from build123d import *

# Parameters (mm, degrees)
SK_PATILLA_R   = 5.1
SK_PATILLA_R_2 = 5
PATILLA_DEPTH  = 8


with BuildPart() as part:
    # Sk_Patilla → Patilla (new body)
    with BuildSketch(Plane.XY.offset(44.4)):
        with BuildLine():
            Line((3.547963542, -28.972606971), (11.45755625, -3.567128365))
            ThreePointArc((11.45755625, -3.567128365), (2.69831408, 11.692694348), (-11.862050632, 1.814319377))
            Line((-11.862050632, 1.814319377), (-15.885042193, -24.488067186))
            ThreePointArc((-15.885042193, -24.488067186), (-8.248595067, -35.743911957), (3.547963542, -28.972606971))
        make_face()
        Circle(SK_PATILLA_R, mode=Mode.SUBTRACT)
        with Locations((-6, -26)):
            Circle(SK_PATILLA_R_2, mode=Mode.SUBTRACT)
    extrude(amount=PATILLA_DEPTH)


solid = part.part
Model file for the job. Use its own axes, mm. Give positions to 0.01 mm unless a question says otherwise; leave off trailing zeros. Loops run counter-clockwise (first coordinate to the right, second up) from the corner with the lowest first, then second, coordinate; pieces in that order, holes last.
Item 1: Slice it at C-C (z = 49.25). Write the cut outline in (x, y), plus the area to 3 significant figures.
Check values:
outline: (-15.89, -24.49) arc R10 ccw to (3.55, -28.97) - (11.46, -3.57) arc R12 ccw (long way) to (-11.86, 1.81) - close; hole circle Ø10 at (-6, -26); hole circle Ø10.2 at (0, 0)
area: 812 mm2
Item 2: Drop a flat-ended pin along its axis: P1, Ø1.5, axis at y = 5.5, z = 49.5, coming from the -X side. Give the stop position or say it passes through.
Check values:
P1: stops at x = -11.02
Item 3: Slice it at D-D (y = -12.5). Write the cut outline in (x, z).
Check values:
outline: (-14.05, 44.4) - (8.68, 44.4) - (8.68, 52.4) - (-14.05, 52.4) - close
Item 4: Drill centre lines: line 1 along Y through (x, z) = (-1.5, 50.25); line 2 along Y through (x, z) = (-6, 49.75); line 3 along Y through (x, z) = (0, 48.75). Where is each one in solid material? Low to high.
Check values:
line 1: y = -34.93 to -28.18, -23.82 to -4.87, 4.87 to 11.91
line 2: y = -36 to -31, -21 to 10.39
line 3: y = -34 to -5.1, 5.1 to 12
Item 5: Mould opens along X. For faces 1 (the face through (-7.08, -30.88, 48.34)), 2 (the face through (-2, -12, 52.4)), 3 (the face through (7.447, -16.448, 48.344)) say: +X half, -X half, draft (parallel to the pull), parting line (faces both ways), or undercut.
Check values:
face 1: undercut
face 2: draft
face 3: +X half
Item 6: Slice it at A-A (x = 0). Write the cut outline in (y, z).
Check values:
outline: (-34, 44.4) - (-5.1, 44.4) - (-5.1, 52.4) - (-34, 52.4) - close; (5.1, 44.4) - (12, 44.4) - (12, 52.4) - (5.1, 52.4) - close
Item 7: Slice it at B-B (y = 0). Write the cut outline in (x, z), plus the area to 3 significant figures.
Check values:
outline: (-12.14, 44.4) - (-5.1, 44.4) - (-5.1, 52.4) - (-12.14, 52.4) - close; (5.1, 44.4) - (12, 44.4) - (12, 52.4) - (5.1, 52.4) - close
area: 112 mm2
